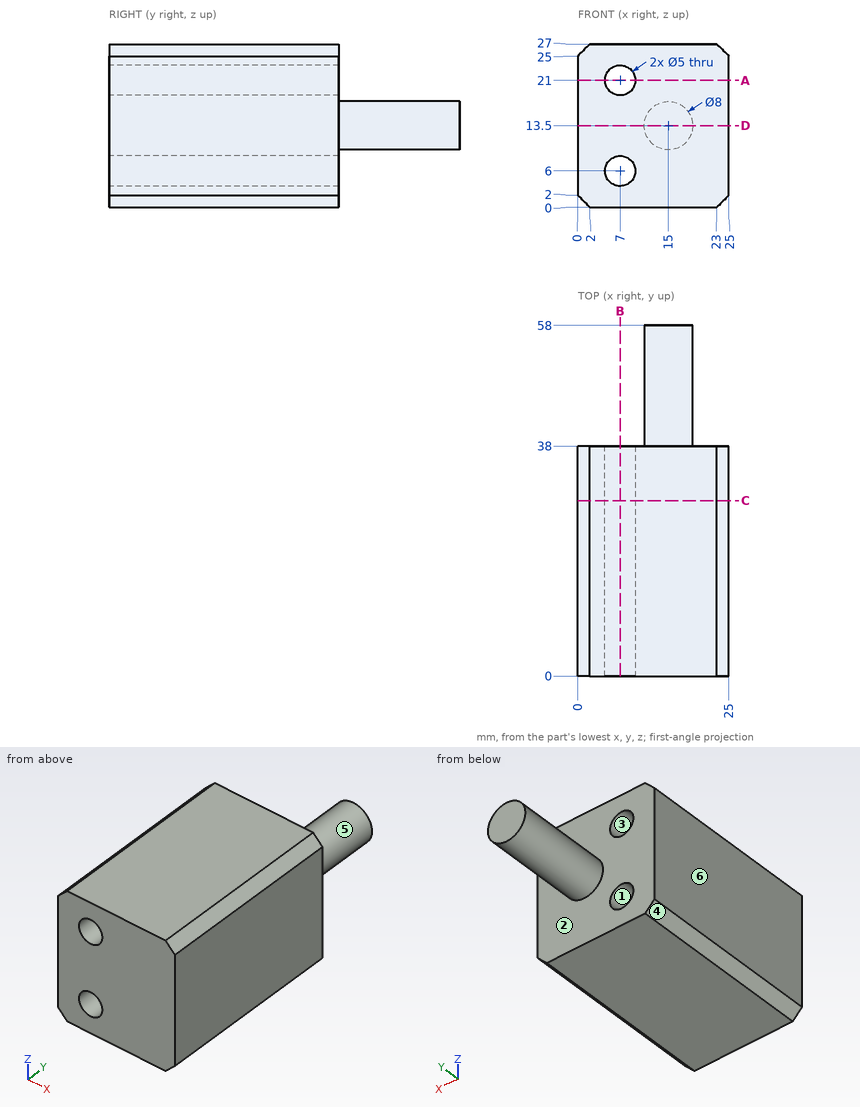
The drawing under review shows one solid part. Ordinate dimensions are in mm from its lowest x, y, z. A direction names the side the tool comes from. Round coordinates to 2 decimals unless told otherwise and drop trailing zeros. Write each loop counter-clockwise with the first axis right and the second up, starting at its lowest first coordinate (ties: lowest second). Pieces come first, ordered by that corner, then holes. Notation, with made-up numbers: (31, 10.25) -> (65, 10.25) arc R30 cw to (65, 44.25) -> close; hole circle Ø9 at (45, -2.75). An arc over 180 degrees is marked (long way). Put each result on its own line as item: value.
Q1. Machinability: for the marked faces 5 and 6, which of the approach directions +Z, -Z, +X, -X, +Y, -Y give a long, thin tool a straight path to every point of the face, cutting with its end or side? Answer none if there is none.
Determined:
face 5: +Y
face 6: +Z, -Z, -X, +Y, -Y
Q2. Clearance check with flat-ended pins moving along their axes: pin 1 Ø12 at (y, z) = (46.5, 4.5) entering from +X; pin 2 Ø4.5 at (x, z) = (7, 6) entering from +Y. State where each tip first meets the part, or that it passes through.
Determined:
pin 1: stops at x = 17.65
pin 2: passes through
Q3. Consider section B-B on x = 7. State the section outline as (y, z) points, and give its area (3 significant figures).
Determined:
outline: (0, 0) -> (38, 0) -> (38, 3.5) -> (0, 3.5) -> close; (0, 8.5) -> (38, 8.5) -> (38, 18.5) -> (0, 18.5) -> close; (0, 23.5) -> (38, 23.5) -> (38, 27) -> (0, 27) -> close
area: 646 mm^2
Q4. Consider section D-D on z = 13.5. State the section outline as (x, y) points, and give its area (3 significant figures).
Determined:
outline: (0, 0) -> (25, 0) -> (25, 38) -> (19, 38) -> (19, 58) -> (11, 58) -> (11, 38) -> (0, 38) -> close
area: 1,110 mm^2
Q5. Consider section A-A on z = 21. State the section outline as (x, y) points.
Determined:
outline: (0, 0) -> (4.5, 0) -> (4.5, 38) -> (0, 38) -> close; (9.5, 0) -> (25, 0) -> (25, 38) -> (9.5, 38) -> close
Q6. Consider section C-C on y = 29. State the section outline as (x, z) points.
Determined:
outline: (0, 2) -> (2, 0) -> (23, 0) -> (25, 2) -> (25, 25) -> (23, 27) -> (2, 27) -> (0, 25) -> close; hole circle Ø5 at (7, 6); hole circle Ø5 at (7, 21)
Q7. To check wall thickness, follow L1, parallel to Z at x = 7, y = 14.5; L2, parallel to Y at x = 3, z = 15.25; L3, parallel to Z at x = 7.5, y = 26.5. State the ranges of each line that lie inside material, in increasing order. Write a range as [from, to].
Determined:
L1: z = [0, 3.5], [8.5, 18.5], [23.5, 27]
L2: y = [0, 38]
L3: z = [0, 3.55], [8.45, 18.55], [23.45, 27]
Q8. The part is to be moulded in two halves that separate along Z. For the marked faces 1, 2, 3 and 4, say which applies: released by +Z, released by -Z, zero draft, split by the parting line, or undercut.
Determined:
face 1: undercut
face 2: zero draft
face 3: undercut
face 4: released by -Z
